Input: part model. Units: mm. Frame: model coordinates. A direction names the side the tool comes from. Give positions to 0.01 mm unless a question says otherwise; leave off trailing zeros. Loops run counter-clockwise (first coordinate to the right, second up) from the corner with the lowest first, then second, coordinate; pieces in that order, holes last. Notation, with made-up numbers: (47.25, -8) - (95.25, -8) arc R11 cw to (95.25, 12) - close; hole circle Ø8 at (81.25, -22.5). An arc over 180 degrees is marked (long way). Answer as a JSON object with one key per item and string values. Group by question number.
(1) Section query C-C (z = 18.5). Return loops of the section in (x, y), plus the area to 3 significant figures.
(2) Section query B-B (x = 6). Return loops of the section in (y, z), plus the area to 3 significant figures.
(3) Section query D-D (x = -40). Return loops of the section in (y, z), plus the area to 3 significant figures.
(4) Section query A-A (z = -6). Return loops of the section in (x, y).
(5) Material intervals for L1, parallel to X at y = 9, z = -1; L2, parallel to X at y = 7.25, z = 52.5; L3, parallel to Z at x = -57.5, y = 2, sorted ascending.
(6) Pin query (flat end, axial travel): P1, Ø3, axis at x = 3, y = 4.5, coming from the +Z side; P2, Ø2, axis at y = 5, z = 62, coming from the -X side; P3, Ø1, axis at x = -36, y = 2, coming from the +Z side. Return the tip coordinate at first contact, or that it passes through.
(7) Mould query, pull axis X, two halves, no side actions, for faces 4 (the flat face through (4, 5, 13.1)), 5 (the cylindrical face through (-47, 5.07, 49.38)), 6 (the flat face through (-10.1, 5, -1)), 7 (the cylindrical face through (-41.73, 4.93, 61.29)). Classes: +X half, -X half, draft (parallel to the pull), parting line (faces both ways), or undercut.
(8) Access query for faces 1 (the flat face through (-13.91, 4.93, 11.08)), 2 (the cylindrical face through (-62.476, 5.07, 73.182)), 3 (the flat face through (-13.1, 5, -2)). Directions: +Z, -Z, +X, -X, +Y, -Y. A direction counts if a zero-diameter tool reaches every point of the face in a straight line with its end or side. Return the directions, or none.
```python
from build123d import *

# Parameters (mm, degrees)
EXTRUDE_1_DEPTH = 10
FILLET_1_R      = 2
FILLET_2_R      = 4


with BuildPart() as part:
    # Эскиз1 → Бобышка-Вытянуть1 (new body)
    with BuildSketch(Plane(origin=(0, 0, 0), x_dir=(1, 0, 0), z_dir=(0, 1, 0))):
        with BuildLine():
            Line((-13.1, 13.1), (-13.1, -6.028932188))
            Line((-13.1, -6.028932188), (-19.160660172, -12.08959236))
            ThreePointArc((-19.160660172, -12.08959236), (-19.160660172, -14.210912703), (-17.039339828, -14.210912703))
            Line((-17.039339828, -14.210912703), (-10.1, -7.271572875))
            Line((-10.1, -7.271572875), (-10.1, 10.1))
            Line((-10.1, 10.1), (10.1, 10.1))
            Line((10.1, 10.1), (10.1, -10.1))
            Line((10.1, -10.1), (-7.271572875, -10.1))
            Line((-7.271572875, -10.1), (-46.997068573, -49.825495698))
            ThreePointArc((-46.997068573, -49.825495698), (-53.506753578, -48.67194049), (-59.415494168, -51.637319575))
            Line((-59.415494168, -51.637319575), (-72.143416229, -64.365241636))
            Line((-72.143416229, -64.365241636), (-66.133008589, -70.375649276))
            Line((-66.133008589, -70.375649276), (-58.516348603, -62.75898929))
            ThreePointArc((-58.516348603, -62.75898929), (-46.687572106, -53.758639918), (-55.687921478, -65.587416415))
            Line((-55.687921478, -65.587416415), (-63.304581464, -73.204076401))
            Line((-63.304581464, -73.204076401), (-57.294173824, -79.214484041))
            Line((-57.294173824, -79.214484041), (-44.566251763, -66.48656198))
            ThreePointArc((-44.566251763, -66.48656198), (-41.600872678, -60.57782139), (-42.754427886, -54.068136385))
            Line((-42.754427886, -54.068136385), (-1.786291501, -13.1))
            Line((-1.786291501, -13.1), (13.1, -13.1))
            Line((13.1, -13.1), (13.1, 13.1))
            Line((13.1, 13.1), (-13.1, 13.1))
        make_face()
    extrude(amount=EXTRUDE_1_DEPTH)

    # Скругление1
    fillet_1_edges = [part.edges().sort_by_distance(p)[0] for p in [
        (10.1, 5, 10.1),
        (10.1, 5, -10.1),
        (-10.1, 5, -10.1),
        (-10.1, 5, 7.271572875),
        (-13.1, 5, 6.028932188),
        (-1.786291501, 5, 13.1),
        (-42.754427886, 5, 54.068136385),
        (-57.294173824, 5, 79.214484041),
        (-63.304581464, 5, 73.204076401),
        (-55.687921478, 5, 65.587416415),
        (-58.516348603, 5, 62.75898929),
        (-66.133008589, 5, 70.375649276),
        (-72.143416229, 5, 64.365241636),
        (-46.997068573, 5, 49.825495698),
        (-7.271572875, 5, 10.1),
    ]]
    fillet(fillet_1_edges, radius=FILLET_1_R)

    # Скругление2
    fillet_2_edges = [part.edges().sort_by_distance(p)[0] for p in [
        (-13.1, 5, -13.1),
        (13.1, 5, -13.1),
        (13.1, 5, 13.1),
    ]]
    fillet(fillet_2_edges, radius=FILLET_2_R)


solid = part.part
```
Recorded:
{
 "1": {"outline": "(-15.67, 0) - (-7.19, 0) - (-7.19, 10) - (-15.67, 10) - close", "area": "84.9 mm^2"},
 "2": {"outline": "(0, -13.1) - (10, -13.1) - (10, -10.1) - (0, -10.1) - close; (0, 10.1) - (10, 10.1) - (10, 13.1) - (0, 13.1) - close", "area": "60.0 mm^2"},
 "3": {"outline": "(0, 42.83) - (10, 42.83) - (10, 51.31) - (0, 51.31) - close", "area": "84.9 mm^2"},
 "4": {"outline": "(-13.1, 0) - (-10.1, 0) - (-10.1, 10) - (-13.1, 10) - close; (10.1, 0) - (13.1, 0) - (13.1, 10) - (10.1, 10) - close"},
 "5": {"L1": "x = -13.1 to -10.1, 10.1 to 13.1", "L2": "x = -60.28 to -55.62, -48.36 to -41.19", "L3": "z = 50.12 to 53.97, 67.4 to 78.38"},
 "6": {"P1": "stops at z = 13.1", "P2": "stops at x = -70.78", "P3": "stops at z = 47.81"},
 "7": {"face 4": "draft", "face 5": "undercut", "face 6": "undercut", "face 7": "+X half"},
 "8": {"face 1": "+Y, -Y", "face 2": "-X, +Y, -Y", "face 3": "-Z, -X, +Y, -Y"}
}
